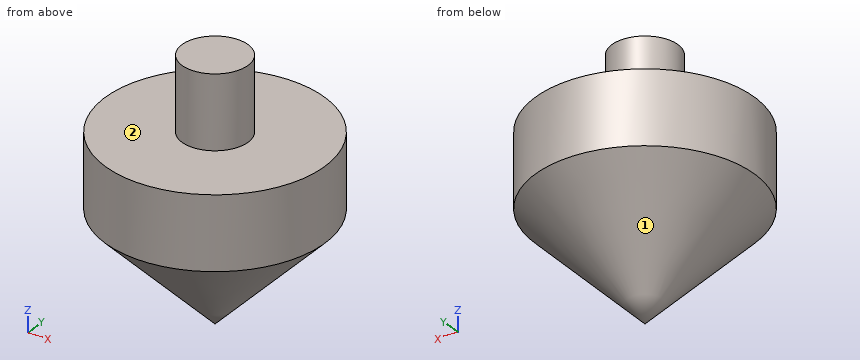
Autodesk Fusion 360 part; units mm, degrees
sketch "Sketch1" plane through (0, 0, 0) normal (0, 0, 1) x (1, 0, 0)
  circle A0 centre (0, 0) radius 15
  dimension "d1" = 30
extrude "Extrude1" add sketch "Sketch1" along normal blind 30
chamfer "Chamfer1" distance 15 angle 45 1 edges at (-13.9849, -5.4242, 0)
extrude "Extrude2" cut 1 faces at (3.8315, 5.6199, 30) along direction (0, 0, -1) blind 5
sketch "Sketch2" plane through (0, 0, 25) normal (0, 0, 1) x (-1, 0, 0)
  circle A0 centre (0, 0) radius 15
  circle A1 centre (0, 0) radius 4.518
  dimension "d7" = 9.036
extrude "Extrude3" add sketch "Sketch2" along normal blind 20 contours A1
extrude "Extrude4" cut 1 faces at (1.3657, -1.8727, 45) along direction (0, 0, -1) blind 10
equation "d7 = ( 4.518 * 2 ) * 1 mm"
The listing builds one solid part. Answer for the finished solid, in the listing's coordinates (mm). Face numbers are marked on the shaded views. A direction names the side the tool comes from. Give positions to 0.01 mm unless a question says otherwise; leave off trailing zeros. Order: outer loops, then holes, each group sorted by start corner. A loop starts at its lowest first (then second) coordinate and runs counter-clockwise, first axis right, second up. Notation, with made-up numbers: (20.25, 2) -> (43.25, 2) arc R27 ccw to (43.25, 29) -> close; hole circle Ø5 at (-34, 40). An arc over 180 degrees is marked (long way). One line per item, written item: value.
1) Find section A-A, the plane z = 4. Determine the outline of the cut face in (x, y).
Reported:
outline: circle Ø8 at (0, 0)
2) Flat-ended cylindrical pins translate along their axes: P1, Ø5, axis at x = 3, y = -3.5, coming from the -Z side; P2, Ø5, axis at x = -5.5, z = 20, coming from the -Y side; P3, Ø8, axis at x = -8.5, y = -2.5, coming from the +Z side; P4, Ø3, axis at x = 1, y = -4.5, coming from the +Z side. Find the tip coordinate at first contact, or state that the pin passes through.
Reported:
P1: stops at z = 2.11
P2: stops at y = -14.7
P3: stops at z = 25
P4: stops at z = 35
3) Find section B-B, the plane z = 26.5. Determine the outline of the cut face in (x, y).
Reported:
outline: circle Ø9.04 at (0, 0)
4) Find the intervals of material crossed by line 1 (Z direction, x = -3, y = -12.25); line 2 (X direction, y = -0.75, z = 14); line 3 (Y direction, x = -2.75, z = 10), in increasing order.
Reported:
line 1: z = 12.61 to 25
line 2: x = -13.98 to 13.98
line 3: y = -9.61 to 9.61
5) A tool of negligible diameter and unlimited length cuts with its end or side. For the marked faces 1 and 2, from which of +Z, -Z, +X, -X, +Y, -Y can it reach the whole face along a straight path? Write none if from no direction.
Reported:
face 1: -Z
face 2: +Z
